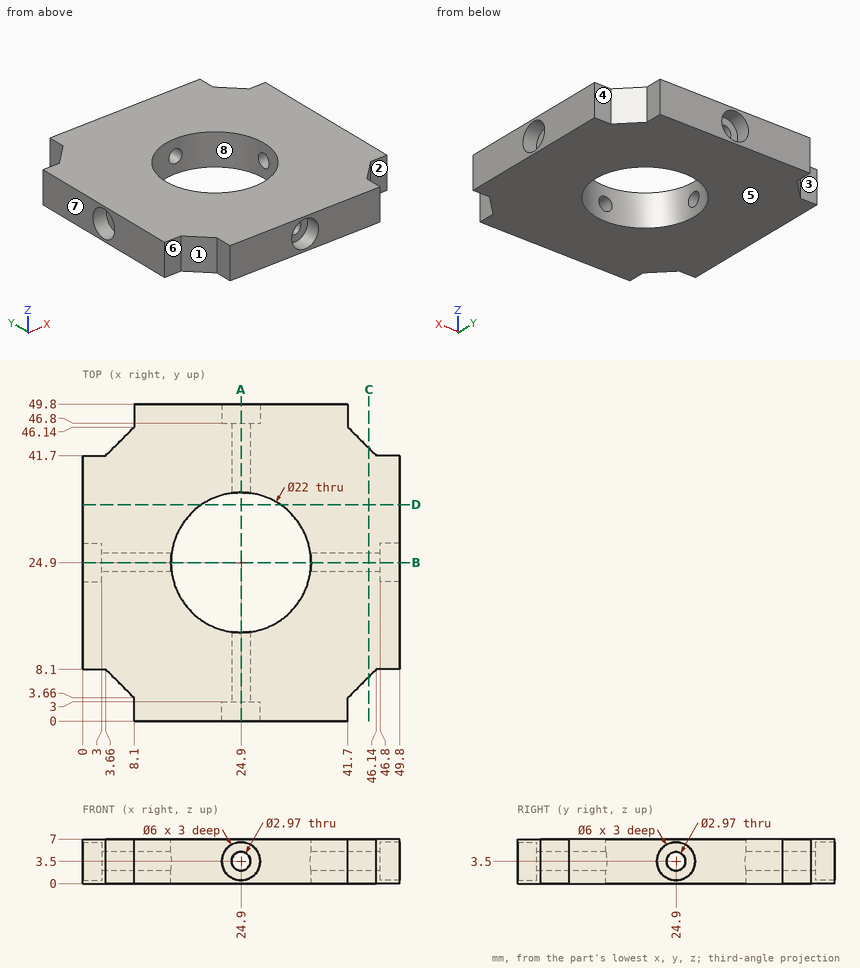
Print and shaded views of the part. All mm, measured from the part's lowest x, y and z. A direction names the side the tool comes from. Round coordinates to 2 decimals unless told otherwise and drop trailing zeros. Write each loop counter-clockwise with the first axis right and the second up, starting at its lowest first coordinate (ties: lowest second). Pieces come first, ordered by that corner, then holes. Notation, with made-up numbers: (40.25, 61) - (79.25, 61) arc R21 ccw to (79.25, 93) - close; hole circle Ø8 at (59, 11.5). An arc over 180 degrees is marked (long way). Use CSV: the item, a comma, the result in double quotes. Start each with the question number.
Item 1: Drill centre lines: L1, parallel to Z at x = 44.75, y = 24.9 (3 decimals); L2, parallel to X at y = 1.1, z = 3.5. Where is each one in solid material? Low to high. Write a range as [from, to].
Item 2: Tool access for the marked faces 1, 2, 3, 4 and 5: list every direction of +Z, -Z, +X, -X, +Y, -Y with a clear straight run to the whole face (end or side of a thin tool).
Item 3: Band-saw the part on A-A (x = 24.9). Write the cut outline in (y, z) (3 decimals).
Item 4: Band-saw the part on C-C (x = 45). Write the cut outline in (y, z) (3 decimals).
Item 5: Two-plate mould, pull along Y, no slides. Class the marked faces 6, 7 and 8: released by +Y, released by -Y, zero draft, split by the parting line, or undercut.
Item 6: Band-saw the part on D-D (y = 34). Write the cut outline in (x, z), and give its area (3 significant figures).
Item 7: Pin check, flat tips, straight feed: P1, Ø3.5, axis at y = 24.9, z = 3.5, coming from the +X side; P2, Ø3, axis at x = 25, z = 3, coming from the +Y side; P3, Ø2, axis at y = 24, z = 6, coming from the -X side; P4, Ø4, axis at y = 24.9, z = 3.5, coming from the -X side. Stop position of each tip, or through.
Checked values:
1,L1,"z = [0, 2.015], [4.985, 7]"
1,L2,"x = [8.1, 21.9], [27.9, 41.7]"
2,face 1,"+Z, -Z, -X, -Y"
2,face 2,"+Z, -Z, +X, -Y"
2,face 3,"+Z, -Z, -X, +Y"
2,face 4,"+Z, -Z, +X, +Y"
2,face 5,"-Z, +X, -X, +Y, -Y"
3,outline,"(0, 0) - (13.9, 0) - (13.9, 2.015) - (3, 2.015) - (3, 0.5) - (0, 0.5) - close; (0, 6.5) - (3, 6.5) - (3, 4.985) - (13.9, 4.985) - (13.9, 7) - (0, 7) - close; (35.9, 0) - (49.8, 0) - (49.8, 0.5) - (46.8, 0.5) - (46.8, 2.015) - (35.9, 2.015) - close; (35.9, 4.985) - (46.8, 4.985) - (46.8, 6.5) - (49.8, 6.5) - (49.8, 7) - (35.9, 7) - close"
4,outline,"(6.96, 0) - (42.84, 0) - (42.84, 7) - (6.96, 7) - close; hole circle Ø2.97 at (24.9, 3.5)"
5,face 6,"released by -Y"
5,face 7,"zero draft"
5,face 8,"undercut"
6,outline,"(0, 0) - (18.72, 0) - (18.72, 7) - (0, 7) - close; (31.08, 0) - (49.8, 0) - (49.8, 7) - (31.08, 7) - close"
6,area,"262 mm²"
7,P1,"stops at x = 46.8"
7,P2,"stops at y = 46.8"
7,P3,"stops at x = 0"
7,P4,"stops at x = 3"
